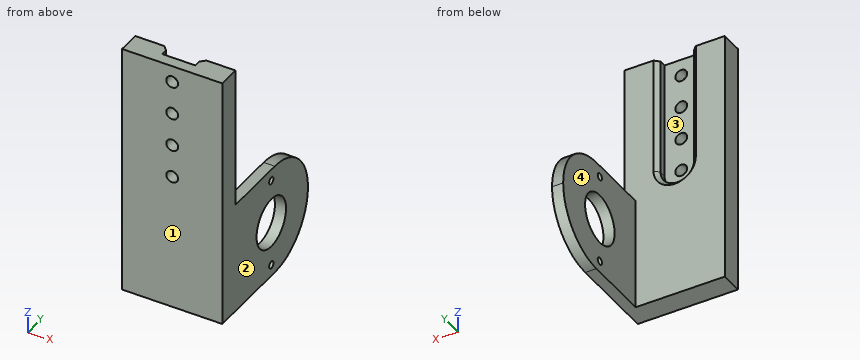
```python
from build123d import *

# Parameters (mm, degrees)
SKETCH1_W           = 57.15
SKETCH1_H           = 145.034
BOSS_EXTRUDE1_DEPTH = 12.7
SKETCH4_R           = 3.3782
CUT_EXTRUDE3_DEPTH  = 157.404199611
CUT_EXTRUDE4_DEPTH  = 6.35
CHAMFER1_SIZE       = 2.54
SKETCH7_W           = 6.35
SKETCH7_H           = 64.008
BOSS_EXTRUDE2_DEPTH = 82.55
SKETCH9_R           = 14.224
SKETCH9_R_2         = 2.032
CUT_EXTRUDE5_DEPTH  = 82.55
FILLET1_R           = 32.004


with BuildPart() as part:
    # Sketch1 → Boss-Extrude1 (new body)
    with BuildSketch(Plane(origin=(0, 0, 0), x_dir=(1, 0, 0), z_dir=(0, 1, 0))):
        with Locations((28.575, 72.517)):
            Rectangle(SKETCH1_W, SKETCH1_H)
    extrude(amount=BOSS_EXTRUDE1_DEPTH)

    # Sketch4 → Cut-Extrude3 (cut, through all)
    with BuildSketch(Plane(origin=(0, 0, 0), x_dir=(-1, 0, 0), z_dir=(0, -1, 0))):
        with Locations(Location((-28.575, 9.525, 0), (0, 0, 90))):
            Circle(SKETCH4_R)
        with Locations(Location((-28.575, 28.575, 0), (0, 0, 90))):
            Circle(SKETCH4_R)
        with Locations(Location((-28.575, 47.625, 0), (0, 0, 90))):
            Circle(SKETCH4_R)
        with Locations(Location((-28.575, 66.675, 0), (0, 0, 90))):
            Circle(SKETCH4_R)
    extrude(amount=-CUT_EXTRUDE3_DEPTH, mode=Mode.SUBTRACT)

    # Sketch8 → Cut-Extrude4 (cut)
    with BuildSketch(Plane(origin=(0, 12.7, 0), x_dir=(1, 0, 0), z_dir=(0, 1, 0))):
        with BuildLine():
            Line((19.05, 66.675), (19.05, 0))
            Line((19.05, 0), (38.1, 0))
            Line((38.1, 0), (38.1, 66.675))
            ThreePointArc((38.1, 66.675), (28.575, 76.2), (19.05, 66.675))
        make_face()
    extrude(amount=-CUT_EXTRUDE4_DEPTH, mode=Mode.SUBTRACT)

    # Chamfer1
    chamfer1_edges = [part.edges().sort_by_distance(p)[0] for p in [
        (28.575, 12.7, -76.2),
        (19.05, 12.7, -33.3375),
        (38.1, 12.7, -33.3375),
    ]]
    chamfer(chamfer1_edges, length=CHAMFER1_SIZE)

    # Sketch7 → Boss-Extrude2 (add)
    with BuildSketch(Plane.XZ):
        with Locations((53.975, -113.03)):
            Rectangle(SKETCH7_W, SKETCH7_H)
    extrude(amount=-BOSS_EXTRUDE2_DEPTH)

    # Sketch9 → Cut-Extrude5 (cut)
    with BuildSketch(Plane.ZY.offset(-50.8)):
        with Locations((-113.03, 47.217289291)):
            Circle(SKETCH9_R)
        with Locations((-87.63, 47.217289291)):
            Circle(SKETCH9_R_2)
        with Locations((-138.43, 47.217289291)):
            Circle(SKETCH9_R_2)
    extrude(amount=-CUT_EXTRUDE5_DEPTH, mode=Mode.SUBTRACT)

    # Fillet1
    fillet1_edges = [part.edges().sort_by_distance(p)[0] for p in [
        (53.975, 82.55, -81.026),
        (53.975, 82.55, -145.034),
    ]]
    fillet(fillet1_edges, radius=FILLET1_R - 0.0001)  # a hair under: the kernel refuses the full size


solid = part.part
```
Geometry check sheet. Reference: the model listing, model coordinates, mm. Face numbers are marked on the shaded views. Coordinates: 2 decimals unless noted, no trailing zeros. Loops run counter-clockwise (first coordinate to the right, second up) from the corner with the lowest first, then second, coordinate; pieces in that order, holes last.
Item 1: Sectioned sample at D-D, the plane y = 40.5. Record the boundary of the cut face in (x, z).
Item 2: Sectioned sample at A-A, the plane y = 54. Record the boundary of the cut face in (x, z).
Item 3: Sectioned sample at C-C, the plane x = 46.5. Record the boundary of the cut face in (y, z).
Item 4: Thickness scan on line 1 (Y direction, x = 55, z = -113); line 2 (X direction, y = 30, z = -93); line 3 (Y direction, x = 6, z = -62). Record the ranges inside material, lowest first.
Item 5: Sectioned sample at B-B, the plane z = -87.63. Record the boundary of the cut face in (x, y).
Item 6: Go/stop test with flat-tipped pins: pin 1 Ø5.5 at (x, z) = (28.575, -28.575) entering from +Y; pin 2 Ø10 at (x, z) = (46, -61) entering from +Y; pin 3 Ø6 at (x, z) = (26, -67) entering from +Y; pin 4 Ø1.9 at (x, y) = (54, 27.5) entering from +Z. Record where each tip stops, or that it passes through.
Item 7: Release check for a two-part mould opening along X. For the marked faces 1, 2, 3 and 4 record: released by +X, released by -X, zero draft, split by the parting line, or undercut.
Check result:
1. outline: (50.8, -145.03) - (57.15, -145.03) - (57.15, -125.57) - (50.8, -125.57) - close; (50.8, -100.49) - (57.15, -100.49) - (57.15, -81.03) - (50.8, -81.03) - close
2. outline: (50.8, -144.85) - (57.15, -144.85) - (57.15, -125.53) - (50.8, -125.53) - close; (50.8, -100.53) - (57.15, -100.53) - (57.15, -81.21) - (50.8, -81.21) - close
3. outline: (0, -145.03) - (12.7, -145.03) - (12.7, 0) - (0, 0) - close
4. line 1: y = 0 to 32.99, 61.44 to 82.55
4. line 2: x = 50.8 to 57.15
4. line 3: y = 0 to 12.7
5. outline: (0, 0) - (57.15, 0) - (57.15, 45.19) - (50.8, 45.19) - (50.8, 12.7) - (0, 12.7) - close; (50.8, 49.25) - (57.15, 49.25) - (57.15, 70.02) - (50.8, 70.02) - close
6. pin 1: passes through
6. pin 2: stops at y = 12.7
6. pin 3: stops at y = 6.35
6. pin 4: stops at z = -81.03
7. face 1: zero draft
7. face 2: released by +X
7. face 3: undercut
7. face 4: released by -X
